Autodesk Inventor part; units mm, degrees
ref_plane "YZ Plane" through (0, 0, 0) normal (1, 0, 0) x (0, 1, 0)
ref_plane "XZ Plane" through (0, 0, 0) normal (0, 1, 0) x (-1, 0, 0)
ref_plane "XY Plane" through (0, 0, 0) normal (0, 0, 1) x (1, 0, 0)
sketch "Sketch1" plane through (0, 0, 0) normal (0, 1, 0) x (-1, 0, 0)
  line L0 (-85.5, 15) -> (0, 15) construction
  line L1 (16, 15) -> (16, -15) construction
  line L2 (16, -15) -> (0, -15) construction
  line L3 (-85.5, -15) -> (-85.5, 15)
  line L4 (16, 0) -> (-42.75, 0) construction
  line L5 (-28.4, 0) -> (23.4, 0) construction
  circle A0 centre (0, 0) radius 11 construction
  line L6 (11, 12.5) -> (11, -13.4099) construction
  circle A1 centre (0, 0) radius 5.05 construction
  line L7 (0, 5.05) -> (7.55, 5.05) construction
  line L8 (0, -5.05) -> (7.55, -5.05) construction
  line L9 (16, 15) -> (16, 5) construction
  line L10 (16, -5) -> (16, -15) construction
  arc A2 (0, 5.05) -> (0, -5.05) centre (0, 0) ccw
  circle A3 centre (0, 0) radius 15 construction
  arc A4 (0, -15) -> (14.1421, -5) centre (0, 0) ccw construction
  arc A5 (14.1421, 5) -> (0, 15) centre (0, 0) ccw construction
  line L11 (0, -15) -> (-85.5, -15) construction
  line L12 (0, 15) -> (16, 15) construction
  arc A6 (11, -8.6603) -> (11, 8.6603) centre (0, 0) ccw construction
  line L13 (-3, -24.7441) -> (-3, 29.6212) construction
  arc A7 (-3, -13.6748) -> (7.55, -11.7897) centre (0, 0) ccw
  line L14 (7.55, 5.05) -> (0, 5.05)
  line L15 (-15, -18.6523) -> (-15, 18.2394) construction
  line L16 (-85.5, -15) -> (-15, -15)
  line L17 (-85.5, 15) -> (-15, 15)
  spline S0 degree 4 poles (-3, -13.6748) (-4.5129, -13.3429) (-7.4407, -12.2328) (-10.459, -15) (-13.4863, -15) (-15, -15) knots 0 0 0 0 0 0.5 1 1 1 1 1
  spline S1 degree 4 poles (-3, 13.6748) (-4.5129, 13.3429) (-7.4407, 12.2328) (-10.459, 15) (-13.4863, 15) (-15, 15) knots 0 0 0 0 0 0.5 1 1 1 1 1
  line L18 (5.05, -20.2789) -> (5.05, 16.2453) construction
  line L19 (7.55, -11.7897) -> (7.55, -5.05)
  line L20 (7.55, 5.05) -> (7.55, 11.7897)
  line L21 (7.55, -5.05) -> (11, -5.05) construction
  line L22 (7.55, 5.05) -> (9.7723, 5.05) construction
  arc A8 (7.55, 11.7897) -> (7.55, -11.7897) centre (0, 0) ccw construction
  arc A9 (7.55, 11.7897) -> (-3, 13.6748) centre (0, 0) ccw
  line L23 (0, -5.05) -> (7.55, -5.05)
  line L24 (0, -35.9242) -> (0, 40.5454) construction
  line L25 (45.18, 0) -> (-107.28, 0)
  line L26 (-42.75, 0) -> (-85.5, 0) construction
  line L27 (-85.5, 0) -> (-44.5655, 0)
  line L28 (-85.5, 0) -> (-37.398, 0)
  line L29 (-37.398, 0) -> (-37.398, -25) construction
  line L30 (-85.5, 15) -> (-85.5, -25) construction
  line L31 (-85.5, -25) -> (-37.398, -25) construction
  point P0 (13.0767, -5)
  point P1 (13.0767, 5)
  dimension "d1" = 22
  dimension "d0" = 30
  dimension "d2" = 85.5
  dimension "d3" = 10.1
  dimension "d4" = 30
  dimension "d5" = 28
  dimension "d6" = 15
  dimension "d7" = 12
  dimension "d8" = 2.5
  dimension "d76" = 48.102
  dimension "d77" = 40
extrude "Extrusion1" add sketch "Sketch1" along normal blind 3
sketch "Sketch2" plane through (0, 3, 0) normal (0, 1, 0) x (1, 0, 0)
  circle A0 centre (0, 0) radius 11 construction
  line L0 (-30.3, 0) -> (104.8, 0) construction
  line L1 (0, 21) -> (0, -21) construction
  line L2 (0, 0) -> (-4.2095, -10.1627) construction
  point P0 (-4.2095, -10.1627)
  point P1 (4.2095, -10.1627)
  point P2 (10.1627, -4.2095)
  point P3 (10.1627, 4.2095)
  point P4 (4.2095, 10.1627)
  point P5 (-4.2095, 10.1627)
  dimension "d19" = 22
  dimension "d20" = 225
  dimension "d78" = 22.5
hole "Hole1" at (-4.2095, 3, 10.1627) at (-4.2095, 3, -10.1627) at (4.2095, 3, -10.1627) at (10.1627, 3, -4.2095) at (10.1627, 3, 4.2095) at (4.2095, 3, 10.1627) direction (0, -1, 0) diameter 2.5 end through all
sketch "Sketch3" plane through (0, 3, 0) normal (0, 1, 0) x (1, 0, 0)
  circle A0 centre (-4.2095, -10.1627) radius 1.25 construction
  circle A1 centre (4.2095, -10.1627) radius 1.25 construction
  circle A2 centre (10.1627, -4.2095) radius 1.25 construction
  circle A3 centre (10.1627, 4.2095) radius 1.25 construction
  circle A4 centre (4.2095, 10.1627) radius 1.25 construction
  circle A5 centre (-4.2095, 10.1627) radius 1.25 construction
  point P0 (0, 0)
sketch "Sketch4" plane through (0, 3, 0) normal (0, 1, 0) x (1, 0, 0)
  line L0 (82.75, -15) -> (82.75, 10.5) construction
  line L1 (85.5, -15) -> (85.5, 15) construction
  line L2 (15, -15) -> (85.5, -15) construction
  point P0 (0, 0)
  point P1 (82.75, -10.5)
  point P2 (82.75, -3.5)
  point P3 (82.75, 3.5)
  dimension "d29" = 2.75
  dimension "d30" = 4.5
  dimension "d33" = 7
hole "Hole2" at (82.75, 3, 10.5) at (82.75, 3, 3.5) at (82.75, 3, -3.5) at (82.75, 3, -10.5) direction (0, -1, 0) diameter 2.5 end through all
sketch "Sketch6" plane through (0, 3, 0) normal (0, 1, 0) x (1, 0, 0)
  line L0 (15, -15) -> (85.5, -15)
  line L1 (80, -15) -> (80, 15)
  line L2 (80, 15) -> (85.5, 15)
  line L3 (85.5, 15) -> (85.5, -15)
  line L4 (85.5, -15) -> (85.5, -15)
  line L5 (80, -15) -> (80, -15)
  line L6 (80, -15) -> (85.5, -15)
  line L7 (85.5, 15) -> (15, 15)
  line L8 (85.5, -15) -> (85.5, 15)
  point P0 (0, 0)
  dimension "d47" = 5.5
extrude "Extrusion2" cut sketch "Sketch6" against normal blind 1
sketch "Sketch7" plane through (0, 3, 0) normal (0, 1, 0) x (1, 0, 0)
  line L0 (-7.55, -13) -> (80, -13) construction
  line L1 (-7.55, 13) -> (80, 13) construction
  line L2 (80, -15) -> (80, 15) construction
  line L3 (80, 15) -> (15, 15) construction
  arc A0 (3, 13.6748) -> (-7.55, 11.7897) centre (0, 0) ccw construction
  line L4 (-7.55, 11.7897) -> (-7.55, 5.05) construction
  line L5 (-7.55, 5.05) -> (0, 5.05) construction
  arc A1 (0, -5.05) -> (0, 5.05) centre (0, 0) ccw construction
  line L6 (0, -5.05) -> (-7.55, -5.05) construction
  line L7 (-7.55, -5.05) -> (-7.55, -11.7897) construction
  arc A2 (-7.55, -11.7897) -> (3, -13.6748) centre (0, 0) ccw construction
  line L8 (15, -15) -> (80, -15) construction
  circle A3 centre (10.1627, -4.2095) radius 1.25 construction
  circle A4 centre (4.2095, 10.1627) radius 1.25 construction
  circle A5 centre (-4.2095, -10.1627) radius 1.25 construction
  circle A6 centre (-4.2095, 10.1627) radius 1.25 construction
  circle A7 centre (10.1627, 4.2095) radius 1.25 construction
  circle A8 centre (4.2095, -10.1627) radius 1.25 construction
  line L9 (30, -13) -> (30, 13) construction
  line L10 (50, -13) -> (50, 13) construction
  line L11 (-7.55, -5.05) -> (-7.55, -11.7897)
  line L12 (-7.55, 11.7897) -> (-7.55, 5.05)
  line L13 (80, -15) -> (80, 15)
  dimension "d50" = 2
  dimension "d51" = 2
  dimension "d52" = 30
  dimension "d53" = 20
hole "Hole3" at (30, 3, 13) at (30, 3, -13) at (50, 3, 13) at (50, 3, -13) direction (0, -1, 0) diameter 3 end through all
sketch "Sketch9" plane through (0, 0, 0) normal (0, -1, 0) x (1, 0, 0)
  circle A0 centre (50, 13) radius 1.5
  circle A1 centre (30, 13) radius 1.5
  circle A2 centre (30, -13) radius 1.5
  circle A3 centre (50, -13) radius 1.5
  circle A4 centre (82.75, -3.5) radius 1.25
  circle A5 centre (82.75, 10.5) radius 1.25
  circle A6 centre (82.75, 3.5) radius 1.25
  circle A7 centre (82.75, -10.5) radius 1.25
  circle A8 centre (10.1627, 4.2095) radius 1.25
  circle A9 centre (4.2095, -10.1627) radius 1.25
  circle A10 centre (-4.2095, 10.1627) radius 1.25
  circle A11 centre (-4.2095, -10.1627) radius 1.25
  circle A12 centre (10.1627, -4.2095) radius 1.25
  circle A13 centre (4.2095, 10.1627) radius 1.25
  line L0 (85.5, -15) -> (85.5, 15)
  line L1 (85.5, 15) -> (15, 15)
  spline S0 degree 4 poles (15, 15) (13.4863, 15) (10.459, 15) (7.4407, 12.2328) (4.5129, 13.3429) (3, 13.6748) knots 0 0 0 0 0 0.5 1 1 1 1 1
  arc A14 (3, 13.6748) -> (-7.55, 11.7897) centre (0, 0) ccw
  line L2 (-7.55, 11.7897) -> (-7.55, 5.05)
  line L3 (-7.55, 5.05) -> (0, 5.05)
  arc A15 (0, -5.05) -> (0, 5.05) centre (0, 0) ccw
  line L4 (0, -5.05) -> (-7.55, -5.05)
  line L5 (-7.55, -5.05) -> (-7.55, -11.7897)
  arc A16 (-7.55, -11.7897) -> (3, -13.6748) centre (0, 0) ccw
  spline S1 degree 4 poles (3, -13.6748) (4.5129, -13.3429) (7.4407, -12.2328) (10.459, -15) (13.4863, -15) (15, -15) knots 0 0 0 0 0 0.5 1 1 1 1 1
  line L6 (15, -15) -> (85.5, -15)
  line L7 (-33.5183, 0) -> (105.3801, 0) construction
  line L8 (53.3261, -18.0641) -> (0.6359, -20.4888)
  spline S2 degree 4 poles (0.6359, -20.4888) (-4.0309, -20.7036) (-10.0323, -18.8785) (-12.1817, -5.2973) (-9.7602, -5.05) (-7.55, -5.05) knots 0 0 0 0 0 0.549784 1 1 1 1 1
  line L9 (15, -15) -> (85.5, -15)
  arc A17 (53.3261, -18.0641) -> (85.5, -15) centre (38.1482, 311.7572) ccw
  line L10 (85.5, 15) -> (15, 15)
  line L11 (-11.2901, -5.05) -> (-3.8099, -5.05) construction
  arc A18 (-4.5618, -5.1264) -> (-10.5382, -5.1264) centre (-7.55, -63.5612) ccw construction
  line L12 (-7.55, -5.05) -> (0, -5.05)
  line L13 (3.8326, -20.3417) -> (-2.5609, -20.6359) construction
  arc A19 (-1.9144, -20.4771) -> (3.1743, -20.2429) centre (-0.5233, 4.7003) ccw construction
  line L14 (0, 5.05) -> (-7.55, 5.05)
  spline S3 degree 4 poles (0.6359, 20.4888) (-4.0309, 20.7036) (-10.0323, 18.8785) (-12.1817, 5.2973) (-9.7602, 5.05) (-7.55, 5.05) knots 0 0 0 0 0 0.549784 1 1 1 1 1
  line L15 (53.3261, 18.0641) -> (0.6359, 20.4888)
  arc A20 (85.5, 15) -> (53.3261, 18.0641) centre (38.1482, -311.7572) ccw
  line L16 (-11.2901, 5.05) -> (-3.8099, 5.05) construction
  arc A21 (-10.5382, 5.1264) -> (-4.5618, 5.1264) centre (-7.55, 63.5612) ccw construction
  line L17 (3.8326, 20.3417) -> (-2.5609, 20.6359) construction
  arc A22 (3.1743, 20.2429) -> (-1.9144, 20.4771) centre (-0.5233, -4.7003) ccw construction
  point P0 (-8.9748, -15.1711)
  point P1 (-10.2976, -6.0407)
  point P2 (-8.9748, 15.1711)
  point P3 (-10.2976, 6.0407)
extrude "Extrusion6" add sketch "Sketch9" against normal blind 3 contours A17 L8 S2 L5 A16 S1 L6 | L1 S0 A14 L2 S3 L15 A20
sketch "Sketch8" plane through (0, 3, 0) normal (0, 1, 0) x (1, 0, 0)
  line L0 (-26.16, 0) -> (104.11, 0) construction
  line L1 (80, -15) -> (80, 15) construction
  line L2 (77, -1.55) -> (80, -1.55)
  line L3 (80, -1.55) -> (80, 1.55)
  line L4 (80, 1.55) -> (77, 1.55)
  line L5 (77, 1.55) -> (77, -1.55) construction
  line L6 (77, -1.55) -> (80, 1.55) construction
  line L7 (80, -1.55) -> (77, 1.55) construction
  arc A0 (77, 1.55) -> (77, -1.55) centre (77, 0) ccw
  point P0 (0, 0)
  point P1 (78.5, 0)
  dimension "d61" = 3
  dimension "d62" = 3.1
extrude "Extrusion3" cut sketch "Sketch8" against normal blind 1
sketch "Sketch10" plane through (0, 2, 0) normal (0, 1, 0) x (1, 0, 0)
  circle A0 centre (82.75, 3.5) radius 1.25
  circle A1 centre (82.75, -10.5) radius 1.25
  circle A2 centre (82.75, -3.5) radius 1.25
  circle A3 centre (82.75, 10.5) radius 1.25
  line L0 (85.5, 15) -> (85.5, -15)
  line L1 (80, 15) -> (85.5, 15)
  line L2 (80, 1.55) -> (80, 15)
  line L3 (77, 1.55) -> (80, 1.55)
  arc A4 (77, 1.55) -> (77, -1.55) centre (77, 0) ccw
  line L4 (80, -1.55) -> (77, -1.55)
  line L5 (80, -15) -> (80, -1.55)
  line L6 (85.5, -15) -> (80, -15)
  line L7 (80, -15) -> (80, -15.7499)
  line L8 (80, -15.7499) -> (85.5, -15.7499)
  line L9 (85.5, 15) -> (85.5, -15)
  line L10 (85.5, -15.7499) -> (85.5, -15)
  line L11 (-31.7181, 0) -> (105.0363, 0) construction
  line L12 (80, 15) -> (80, 15.7499)
  line L13 (80, 15.7499) -> (85.5, 15.7499)
  line L14 (85.5, 15.7499) -> (85.5, 15)
  arc A5 (53.3261, -18.0641) -> (85.5, -15) centre (38.1482, 311.7572) ccw
  point P0 (0, 0)
extrude "Extrusion7" cut sketch "Sketch10" along normal blind 1 contours L1 L12 L13 L14 | A5 L7 L6 | L10 L8 A5
ref_plane "Work Plane1" through (-10.6877, 1.5, -8.1148) normal (-1, 0, 0) x (0, -1, 0)
equation "\"d3\" = d12 + diameter_tol"
equation "\"d19\" = d21"
equation "\"d29\" = hole_2_bottom"
equation "\"d47\" = border_thickness"
equation "\"d10\" = 22"
equation "\"d12\" = 10"
equation "\"d14\" = 2 * d13"
equation "\"base_width\" = 6.25"
equation "\"d21\" = 22"
equation "\"diameter_tol\" = 0.1"
equation "\"border_thickness\" = 5.5"
equation "\"hole_2_bottom\" = 2.75"
properties part number "new_side_u106_long_design" material "Aluminum 2014-T4"
Check sheet for the modelled part. Datum: model origin and axes. Units: mm. A direction names the side the tool comes from. Round coordinates to 2 decimals unless told otherwise and drop trailing zeros. Order: outer loops, then holes, each group sorted by start corner. A loop starts at its lowest first (then second) coordinate and runs counter-clockwise, first axis right, second up. Notation, with made-up numbers: (-6.75, 12.5) -> (41.25, 12.5) arc R25 cw to (41.25, 27.5) -> close; hole circle Ø1 at (23, 52.25). An arc over 180 degrees is marked (long way). Use CSV: the item, a comma, the result in double quotes.
(1) Cross-section at B-B (x = 50). Record the boundary of the cut face in (y, z), and give its area (3 significant figures).
Worked out:
outline,"(0, -18.22) -> (3, -18.22) -> (3, -14.5) -> (0, -14.5) -> close; (0, -11.5) -> (3, -11.5) -> (3, 11.5) -> (0, 11.5) -> close; (0, 14.5) -> (3, 14.5) -> (3, 18.22) -> (0, 18.22) -> close"
area,"91.3 mm²"
(2) Depth check by flat-ended pin: pin 1 (1 mm diameter, centred on x = 49.5, y = 1, fed in from +Z); pin 2 (1.5 mm diameter, centred on x = 66.5, z = -1.5, fed in from -Y); pin 3 (3 mm diameter, centred on x = 82.75, z = 10.5, fed in from +Y). Enter the tip coordinate at first touch or a pass-through.
Worked out:
pin 1,"z = 18.26"
pin 2,"y = 0"
pin 3,"y = 2"
(3) Tool access check on faces 4 (the face through (-4, 1, 5.05)), 5 (the face through (27.35, 1.48, 19.26)). Record the directions out of +Z, -Z, +X, -X, +Y, -Y that give a thin tool (end or side, any length) a straight path to the whole face; none if there is none.
Worked out:
face 4,"-X, +Y, -Y"
face 5,"+Z, +X, +Y, -Y"
(4) Cross-section at A-A (x = 82.75). Record the boundary of the cut face in (y, z).
Worked out:
outline,"(0, -15.39) -> (2, -15.39) -> (2, -11.75) -> (0, -11.75) -> close; (0, -9.25) -> (2, -9.25) -> (2, -4.75) -> (0, -4.75) -> close; (0, -2.25) -> (2, -2.25) -> (2, 2.25) -> (0, 2.25) -> close; (0, 4.75) -> (2, 4.75) -> (2, 9.25) -> (0, 9.25) -> close; (0, 11.75) -> (2, 11.75) -> (2, 15.39) -> (0, 15.39) -> close"
(5) Draft check along Z on faces 1 (the face through (27.35, 1.48, -19.26)), 2 (the face through (3.155, 1.479, 10.835)), 3 (the face through (85.5, 1, 0)). Enter one of: pulls with the +Z half, pulls with the -Z half, needs draft (parallel to the pull), parting line crosses it, or undercut.
Worked out:
face 1,"pulls with the -Z half"
face 2,"undercut"
face 3,"needs draft"
(6) Cross-section at D-D (x = 39.5). Record the boundary of the cut face in (y, z), and give its area (3 significant figures).
Worked out:
outline,"(0, -18.7) -> (3, -18.7) -> (3, 18.7) -> (0, 18.7) -> close"
area,"112 mm²"
(7) Material ranges on line 1 along Z through (x, y) = (31, 0.35); line 2 along X through (y, z) = (2.3, -13); line 3 along Z through (x, y) = (82.75, 0.4), recorded low to high. Write a range as from..to.
Worked out:
line 1,"-19.09..-14.12, -11.88..11.88, 14.12..19.09"
line 2,"-9.84..28.5, 31.5..48.5, 51.5..80"
line 3,"-15.39..-11.75, -9.25..-4.75, -2.25..2.25, 4.75..9.25, 11.75..15.39"
(8) Cross-section at C-C (z = -10.5). Count the separate pieces of the cut face and the enclosed holes in it, and give its area (3 significant figures).
Worked out:
separate pieces,"4"
enclosed holes,"0"
area,"263 mm²"
